Geometry: final body of the model. Coordinates: model frame, mm. Coordinates: 2 decimals unless noted, no trailing zeros. Order: outer loops, then holes, each group sorted by start corner. A loop starts at its lowest first (then second) coordinate and runs counter-clockwise, first axis right, second up. Notation, with made-up numbers: (-33, -31.75) -> (-1, -31.75) arc R6 cw to (-1, -27.75) -> close; hole circle Ø10 at (10.25, 80). An arc over 180 degrees is marked (long way). Answer in a Markdown table with one row per item. Add a question column.
1) Ray query, line 1 (X direction, y = 2.75, z = -15.5); line 2 (Y direction, x = -0.25, z = -22). Return the intervals inside material, ascending. Write a range as from..to.
2) Section query D-D on x = -0.25. Return the cut outline in (y, z), then the cut area to 3 significant figures.
3) Section query C-C on x = 3.25. Return the cut outline in (y, z), then the cut area to 3 significant figures.
4) Contact query for flat-ended pins moving along their axis: P1, Ø1, axis at x = 5.5, z = -4.5, coming from the +Y side; P2, Ø1, axis at x = 4, y = 2, coming from the +Z side; P3, Ø2, axis at y = 0.5, z = 10.5, coming from the +X side. Output: stop coordinate, or through.
5) Section query A-A on x = -3.25. Return the cut outline in (y, z), then the cut area to 3 significant figures.
6) Section query B-B on z = -11. Return the cut outline in (x, y).
```python
from build123d import *

# Parameters (mm, degrees)
EXTRUSION1_DEPTH             = 38
ENL_V_MAT_EXTRU_1_DEPTH      = 77
R_P_TITION_CIRCULAIRE1_COUNT = 2
R_P_TITION_CIRCULAIRE1_ANGLE = 90


with BuildPart() as part:
    # Esquisse1 → Extrusion1 (new body, symmetric)
    with BuildSketch(Plane.XY):
        with BuildLine():
            Line((-6, 5), (-6, -5))
            ThreePointArc((-6, -5), (-5.707106781, -5.707106781), (-5, -6))
            Line((-5, -6), (5, -6))
            ThreePointArc((5, -6), (5.707106781, -5.707106781), (6, -5))
            Line((6, -5), (6, 5))
            ThreePointArc((6, 5), (5.707106781, 5.707106781), (5, 6))
            Line((5, 6), (-5, 6))
            ThreePointArc((-5, 6), (-5.707106781, 5.707106781), (-6, 5))
        make_face()
    extrude(amount=EXTRUSION1_DEPTH, both=True)

    # Esquisse3 → Enl_v. mat.-Extru.1 (cut, through all)
    with BuildSketch(Plane.XY.offset(38)):
        Polygon((6, 2), (4.8, 2), (4.8, 4), (2, 1), (2, -1), (4.8, -4), (4.8, -2), (6, -2), align=None)
    enl_v_mat_extru_1 = extrude(amount=-ENL_V_MAT_EXTRU_1_DEPTH, mode=Mode.SUBTRACT)

    # R_p_tition circulaire1: Enl_v. mat.-Extru.1 ×2 about axis
    r_p_tition_circulaire1_axis = Axis((0, 0, 0), (0, 0, 1))
    for i in range(1, R_P_TITION_CIRCULAIRE1_COUNT):
        add(enl_v_mat_extru_1.rotate(r_p_tition_circulaire1_axis, i * R_P_TITION_CIRCULAIRE1_ANGLE / (R_P_TITION_CIRCULAIRE1_COUNT - 1)), mode=Mode.SUBTRACT)


solid = part.part
```
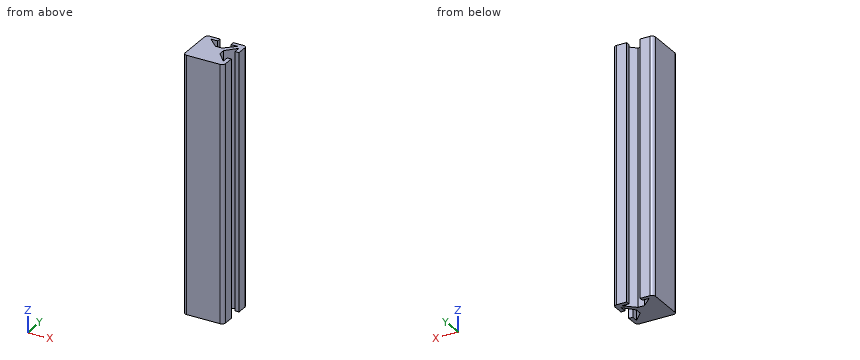
Result:
| question | item | result |
|---|---|---|
| 1 | line 1 | -6..-1.8, 1.8..3.63, 4.8..6 |
| 1 | line 2 | -6..2 |
| 2 | outline | (-6, -38) -> (2, -38) -> (2, 38) -> (-6, 38) -> close |
| 2 | area | 608 mm2 |
| 3 | outline | (-6, -38) -> (-2.34, -38) -> (-2.34, 38) -> (-6, 38) -> close; (2.34, -38) -> (4.1, -38) -> (4.1, 38) -> (2.34, 38) -> close; (4.8, -38) -> (6, -38) -> (6, 38) -> (4.8, 38) -> close |
| 3 | area | 503 mm2 |
| 4 | P1 | y = 6 |
| 4 | P2 | through |
| 4 | P3 | x = 2.47 |
| 5 | outline | (-6, -38) -> (4.1, -38) -> (4.1, 38) -> (-6, 38) -> close; (4.8, -38) -> (6, -38) -> (6, 38) -> (4.8, 38) -> close |
| 5 | area | 859 mm2 |
| 6 | outline | (-6, -5) arc R1 ccw to (-5, -6) -> (5, -6) arc R1 ccw to (6, -5) -> (6, -2) -> (4.8, -2) -> (4.8, -4) -> (2, -1) -> (2, 1) -> (4.8, 4) -> (4.8, 2) -> (6, 2) -> (6, 5) arc R1 ccw to (5, 6) -> (2, 6) -> (2, 4.8) -> (4, 4.8) -> (1, 2) -> (-1, 2) -> (-4, 4.8) -> (-2, 4.8) -> (-2, 6) -> (-5, 6) arc R1 ccw to (-6, 5) -> close |
